The figure shows three views and two pictorial views of one solid part (mm, origin at its lowest corner). Answer the questions. Round coordinates to 2 decimals unless told otherwise and drop trailing zeros. Order: outer loops, then holes, each group sorted by start corner. A loop starts at its lowest first (then second) coordinate and runs counter-clockwise, first axis right, second up. Notation, with made-up numbers: (68.25, -11.75) -> (82.25, -11.75) arc R22 ccw to (82.25, 8.25) -> close; hole circle Ø10 at (6, 81). An arc over 180 degrees is marked (long way). One line per item, written item: value. Start each with the question number.
1. Section B-B (z = 0.55) is taken. Give the vertices of the cut face in (x, y) (1 decimal).
2. Flat-ended cylindrical pins translate along their axes: pin 1 Ø4.5 at (x, y) = (15.11, 100.25) entering from -Z; pin 2 Ø1 at (x, z) = (16.5, 0.5) entering from -Y. Find the tip coordinate at first contact, or state that the pin passes through.
3. Section A-A (x = 15) is taken. Give the vertices of the cut face in (y, z).
4. Consider line 1 (X direction, y = 10, z = 1.2); line 2 (Y direction, x = 19, z = 1.05); line 3 (Y direction, x = 16, z = 0.4) (1 decimal). Determine where each line is inside the solid, lowest interval first.
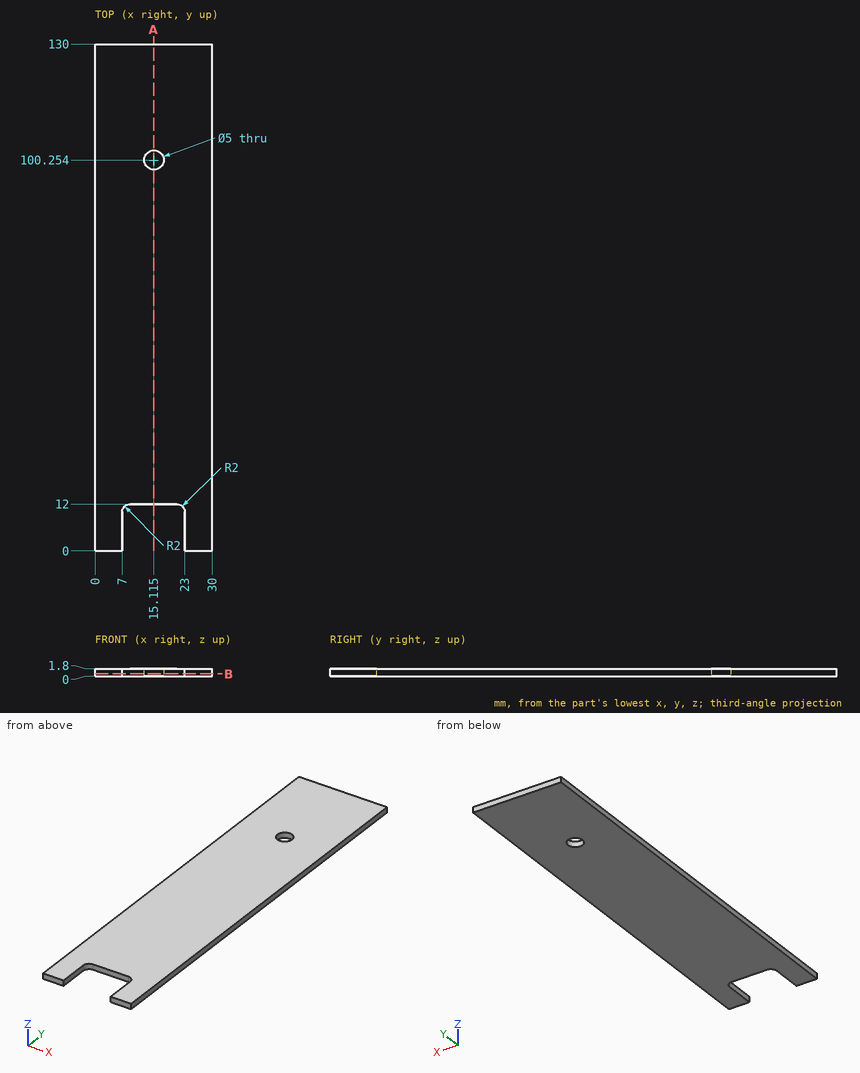
Answer:
1. outline: (0, 0) -> (7, 0) -> (7, 10) arc R2 cw to (9, 12) -> (21, 12) arc R2 cw to (23, 10) -> (23, 0) -> (30, 0) -> (30, 130) -> (0, 130) -> close; hole circle Ø5 at (15.1, 100.3)
2. pin 1: through
2. pin 2: y = 12
3. outline: (12, 0) -> (97.76, 0) -> (97.76, 1.8) -> (12, 1.8) -> close; (102.75, 0) -> (130, 0) -> (130, 1.8) -> (102.75, 1.8) -> close
4. line 1: 0 to 7, 23 to 30
4. line 2: 12 to 130
4. line 3: 12 to 97.9, 102.6 to 130
